```python
from build123d import *

# Parameters (mm, degrees)
SKETCH3_R           = 10
BOSS_EXTRUDE1_DEPTH = 10
SKETCH3_5_R         = 10
SKETCH3_5_R_2       = 5
BOSS_EXTRUDE3_DEPTH = 5


with BuildPart() as part:
    # Sketch3 → Boss-Extrude1 (new body)
    with BuildSketch(Plane(origin=(0, 0, 0), x_dir=(1, 0, 0), z_dir=(0, 1, 0))):
        with BuildLine():
            Line((-31.848796088, 25), (-26.723993282, 25))
            Line((-26.723993282, 25), (-26.723993282, 40))
            ThreePointArc((-26.723993282, 40), (-11.848796088, 54.875197195), (3.026401107, 40))
            Line((3.026401107, 40), (3.026401107, 15))
            Line((3.026401107, 15), (58.151203912, 15))
            ThreePointArc((58.151203912, 15), (73.151203912, 0), (58.151203912, -15))
            Line((58.151203912, -15), (3.026401107, -15))
            Line((3.026401107, -15), (3.026401107, -40))
            ThreePointArc((3.026401107, -40), (-11.848796088, -54.875197195), (-26.723993282, -40))
            Line((-26.723993282, -40), (-26.723993282, -25))
            Line((-26.723993282, -25), (-31.848796088, -25))
            ThreePointArc((-31.848796088, -25), (-42.455397805, -20.606601718), (-46.848796088, -10))
            Line((-46.848796088, -10), (-46.848796088, 10))
            ThreePointArc((-46.848796088, 10), (-42.455397805, 20.606601718), (-31.848796088, 25))
        make_face()
        with Locations(Location((-11.848796088, -40, 0), (0, 0, 270))):
            Circle(SKETCH3_R, mode=Mode.SUBTRACT)
        with Locations(Location((-11.848796088, 40, 0), (0, 0, 270))):
            Circle(SKETCH3_R, mode=Mode.SUBTRACT)
        with Locations(Location((58.151203912, 0, 0), (0, 0, 270))):
            Circle(SKETCH3_R, mode=Mode.SUBTRACT)
        with BuildLine():
            ThreePointArc((-39.348796088, -10), (-31.848796088, -17.5), (-24.348796088, -10))
            Line((-24.348796088, -10), (-24.348796088, 10))
            ThreePointArc((-24.348796088, 10), (-31.848796088, 17.5), (-39.348796088, 10))
            Line((-39.348796088, 10), (-39.348796088, -10))
        make_face(mode=Mode.SUBTRACT)
    extrude(amount=BOSS_EXTRUDE1_DEPTH)

    # Sketch3_5 → Boss-Extrude3 (add)
    # profile 1 of 3: a face of its own
    with BuildSketch(Plane(origin=(0, 0, 0), x_dir=(1, 0, 0), z_dir=(0, 1, 0))):
        with Locations(Location((-11.848796088, 40, 0), (0, 0, 270))):
            Circle(SKETCH3_5_R)
        with Locations(Location((-11.848796088, 40, 0), (0, 0, 270))):
            Circle(SKETCH3_5_R_2, mode=Mode.SUBTRACT)
    # profile 2 of 3: a face of its own
    with BuildSketch(Plane(origin=(0, 0, 0), x_dir=(1, 0, 0), z_dir=(0, 1, 0))):
        with Locations(Location((-11.848796088, -40, 0), (0, 0, 270))):
            Circle(SKETCH3_5_R)
        with Locations(Location((-11.848796088, -40, 0), (0, 0, 270))):
            Circle(SKETCH3_5_R_2, mode=Mode.SUBTRACT)
    # profile 3 of 3: a face of its own
    with BuildSketch(Plane(origin=(0, 0, 0), x_dir=(1, 0, 0), z_dir=(0, 1, 0))):
        with Locations(Location((58.151203912, 0, 0), (0, 0, 270))):
            Circle(SKETCH3_5_R)
        with Locations(Location((58.151203912, 0, 0), (0, 0, 270))):
            Circle(SKETCH3_5_R_2, mode=Mode.SUBTRACT)
    extrude(amount=BOSS_EXTRUDE3_DEPTH)


solid = part.part
```
Geometry check sheet. Reference: the model listing, model coordinates, mm. A direction names the side the tool comes from. Round coordinates to 2 decimals unless told otherwise and drop trailing zeros. Loops run counter-clockwise (first coordinate to the right, second up) from the corner with the lowest first, then second, coordinate; pieces in that order, holes last. Notation, with made-up numbers: (-15, 67.5) - (30, 67.5) arc R30 ccw to (30, 99.5) - close; hole circle Ø5 at (78, 82). An arc over 180 degrees is marked (long way). Write each question's results on one line, items separated by ' | '. Start each with the question number.
Q1. Cross-section at C-C on z = 38. Enter the section's corners in (x, y).
Q2. Release check for a two-part mould opening along Z. For faces 1 (the flat face through (3.026, 5, -28)), 2 (the flat face through (-29, 5, 25)), 3 (the cylindrical face through (66.58, 7.46, 5.38)) record: +Z half, -Z half, draft (parallel to the pull), parting line (faces both ways), or undercut.
Q3. Access from +Z, -Z, +X, -X, +Y, -Y to the whole of each face (thin tool, end or side, straight path). Record for faces 4 (the flat face through (3.026, 5, 27)), 5 (the flat face through (30, 5, -15)), 6 (the flat face through (63, 5, 2)).
Q4. Thickness scan on line 1 (X direction, y = 8.95, z = 0); line 2 (Z direction, x = -10.5, y = 2.5); line 3 (X direction, y = 5.25, z = -39.5). Record the ranges inside material, lowest first. Write a range as [from, to].
Q5. Cross-section at B-B on x = 61. Enter the section's corners in (y, z).
Q6. Gauge pin test, flat ends, axial feed: P1, Ø3, axis at y = 7, z = 17.5, coming from the +X side; P2, Ø3, axis at y = 5, z = -32, coming from the -X side; P3, Ø16, axis at x = -11.85, z = -40, coming from the +Y side. Record the tip position at first contact, or that the pin passes through.
Q7. Cross-section at A-A on z = 0. Enter the section's corners in (x, y).
Answers below:
1) outline: (-26.72, 0) - (-16.43, 0) - (-16.43, 5) - (-21.65, 5) - (-21.65, 10) - (-26.72, 10) - close; (-7.27, 0) - (3.03, 0) - (3.03, 10) - (-2.05, 10) - (-2.05, 5) - (-7.27, 5) - close
2) face 1: draft | face 2: +Z half | face 3: undercut
3) face 4: +Z, +X, +Y, -Y | face 5: -Z, +X, +Y, -Y | face 6: +Y
4) line 1: x = [-46.85, -39.35], [-24.35, 48.15], [68.15, 73.15] | line 2: z = [-54.81, -44.81], [-35.19, 35.19], [44.81, 54.81] | line 3: x = [-26.72, -21.84], [-1.86, 3.03]
5) outline: (0, -14.73) - (10, -14.73) - (10, -9.59) - (5, -9.59) - (5, -4.11) - (0, -4.11) - close; (0, 4.11) - (5, 4.11) - (5, 9.59) - (10, 9.59) - (10, 14.73) - (0, 14.73) - close
6) P1: stops at x = 3.03 | P2: stops at x = -26.72 | P3: stops at y = 5
7) outline: (-46.85, 0) - (-39.35, 0) - (-39.35, 10) - (-46.85, 10) - close; (-24.35, 0) - (53.15, 0) - (53.15, 5) - (48.15, 5) - (48.15, 10) - (-24.35, 10) - close; (63.15, 0) - (73.15, 0) - (73.15, 10) - (68.15, 10) - (68.15, 5) - (63.15, 5) - close
